Geometry check sheet. Reference: the model listing, model coordinates, mm. Face numbers are marked on the shaded views. A direction names the side the tool comes from. Coordinates: 2 decimals unless noted, no trailing zeros. Order: outer loops, then holes, each group sorted by start corner. A loop starts at its lowest first (then second) coordinate and runs counter-clockwise, first axis right, second up. Notation, with made-up numbers: M 65.25,35.25 L 117.25,35.25 A25 cw 117.25,67.25 Z; hole C 45,52 d6. An arc over 180 degrees is marked long. One line per item, written item: value. Start each with the question number.
1) Thickness scan on L1, parallel to X at y = -21, z = -62.5; L2, parallel to Y at x = 45, z = -100.5; L3, parallel to Z at x = -42, y = 38. Record the ranges inside material, lowest first. Write a range as from..to.
2) Sectioned sample at D-D, the plane y = -38.5. Enter the section's corners in (x, z), then the cut area to 3 significant figures.
3) Sectioned sample at A-A, the plane x = 20. Enter the section's corners in (y, z), then the cut area to 3 significant figures.
4) Go/stop test with flat-tipped pins: P1, Ø1, axis at x = -15.5, z = -83, coming from the +Y side; P2, Ø5, axis at x = -25.5, z = -82, coming from the -Y side. Record where each tip stops, or that it passes through.
5) Access from +Z, -Z, +X, -X, +Y, -Y to the whole of each face (thin tool, end or side, straight path). Record for the marked faces 1, 2 and 3.
6) Sectioned sample at B-B, the plane y = -10. Enter the section's corners in (x, z), then the cut area to 3 significant figures.
7) Sectioned sample at C-C, the plane z = -71.5. Enter the section's corners in (x, y), then the cut area to 3 significant figures.
```python
from build123d import *

# Parameters (mm, degrees)
F0_W     = 127
F0_H     = 63.5
F1_DEPTH = 50.8
F3_D     = 5.4102
F3_DEPTH = 12.7
F3_TIP   = 1.6253880605
F6_W     = 89.9240933359
F6_H     = 71.2126605213
F5_DEPTH = 132.9497303814
F7_R     = 5


with BuildPart() as f1:
    # F0 (on Front) → F1 (new body, symmetric)
    with BuildSketch(Plane.XZ):
        with Locations((11.2671367824, -14.1953701283)):
            Rectangle(F0_W, F0_H)
    extrude(amount=F1_DEPTH, both=True)

    # F3
    with Locations(Plane.XY.offset(17.5546298717)):
        with Locations((4.0161549114, 7.0065222681)):
            Hole(F3_D / 2, depth=F3_DEPTH)
            with Locations((0, 0, -(F3_DEPTH + F3_TIP / 2))):  # 118° drill point
                Cone(0, F3_D / 2, F3_TIP, mode=Mode.SUBTRACT)

    # F6 (on face) → F5 (join)
    with BuildSketch(Plane(origin=(0, 0, -45.9453701283), x_dir=(1, 0, 0), z_dir=(0, 0, -1))):
        with Locations((20.2872846276, -7.0287231356)):
            Rectangle(F6_W, F6_H)
    extrude(amount=F5_DEPTH)

    # F7
    f7_edges = [f1.edges().sort_by_distance(p)[0] for p in [
        (74.767137, 50.8, -14.19537),
        (-52.232863, 50.8, -14.19537),
    ]]
    fillet(f7_edges, radius=F7_R)


solid = f1.part
```
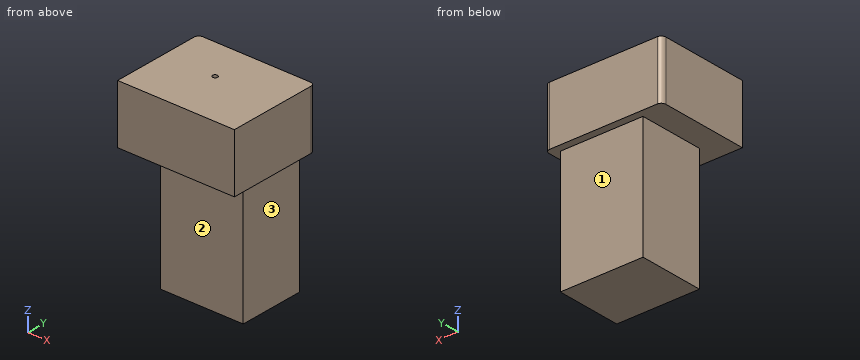
Final values:
1. L1: x = -24.67..65.25
1. L2: y = -28.58..42.64
1. L3: z = -45.95..17.55
2. outline: M -52.23,-45.95 L 74.77,-45.95 L 74.77,17.55 L -52.23,17.55 Z
2. area: 8,060 mm^2
3. outline: M -50.8,-45.95 L -28.58,-45.95 L -28.58,-178.9 L 42.64,-178.9 L 42.64,-45.95 L 50.8,-45.95 L 50.8,17.55 L -50.8,17.55 Z
3. area: 15,900 mm^2
4. P1: stops at y = 42.64
4. P2: stops at y = -28.58
5. face 1: -Z, +X, -X, +Y
5. face 2: -Z, +X, -X, -Y
5. face 3: -Z, +X, +Y, -Y
6. outline: M -52.23,-45.95 L -24.67,-45.95 L -24.67,-178.9 L 65.25,-178.9 L 65.25,-45.95 L 74.77,-45.95 L 74.77,17.55 L -52.23,17.55 Z
6. area: 20,000 mm^2
7. outline: M -24.67,-28.58 L 65.25,-28.58 L 65.25,42.64 L -24.67,42.64 Z
7. area: 6,400 mm^2
